Model file for the job. Use its own axes, mm. A direction names the side the tool comes from. Give positions to 0.01 mm unless a question says otherwise; leave off trailing zeros. Loops run counter-clockwise (first coordinate to the right, second up) from the corner with the lowest first, then second, coordinate; pieces in that order, holes last. Notation, with made-up numbers: (16, 1.25) - (39, 1.25) arc R20 ccw to (39, 31.25) - close; hole circle Ø7 at (0, 89). An arc over 180 degrees is marked (long way). Answer as CSV lines item,"result". Start each with the question number.
Item 1: Drill centre lines: L1, parallel to Y at x = 575, z = 109; L2, parallel to Z at x = 522.5, y = 36.5; L3, parallel to X at y = 82.5, z = 88. Where is each one in solid material? Low to high. Write a range as from..to.
Item 2: Pin check, flat tips, straight feed: pin 1 (5 mm diameter, centred on x = 640.5, z = 101.5, fed in from +Y); pin 2 (10 mm diameter, centred on y = 115.5, z = 57, fed in from -X); pin 3 (5 mm diameter, centred on y = 26.5, z = 36.5, fed in from +X). Stop position of each tip, or through.
Item 3: Saw through at D-D on y = 101.5. Give the cut face in (x, z), plus the area to 3 significant figures.
Item 4: Pull direction X, two halves, no side cores. Call faces 1 (the flat face through (609.33, 88.2, 59.16)), 2 (the flat face through (645, 94, 64)), 3 (the flat face through (591, 28, 130)): pulls with the +X half, pulls with the -X half, needs draft (parallel to the pull), parting line crosses it, or undercut.
Item 5: Saw through at B-B on z = 59. Give the cut face in (x, y), plus the area to 3 significant figures.
Item 6: Tool access for faces 4 (the flat face through (550, 50, 64)), 5 (the cylindrical face through (600.02, 0.88, 125.07)), 6 (the cylindrical face through (659.11, -8.4, 59.16)), 7 (the flat face through (588, 10, 120)): list every direction of +Z, -Z, +X, -X, +Y, -Y with a clear straight run to the whole face (end or side of a thin tool).
Item 7: Saw through at A-A on y = 0. Give the cut face in (x, z), plus the area to 3 significant figures.
Item 8: Saw through at C-C on x = 567. Give the cut face in (y, z), plus the area to 3 significant figures.
from build123d import *

# Parameters (mm, degrees)
EXTRUDE_1_DEPTH     = 130
SHELL_2_T           = -10
SKETCH_2_W          = 10
SKETCH_2_H          = 80.0247511
CUT_EXTRUDE_1_DEPTH = 120
SKETCH_3_R          = 20
CUT_EXTRUDE_2_DEPTH = 10


with BuildPart() as part:
    # 草图1 → 凸台-拉伸1 (new body)
    with BuildSketch(Plane.XY):
        with BuildLine():
            Line((574.017492235, -50), (620, -50))
            ThreePointArc((620, -50), (668.296291314, -12.940952255), (645, 43.301270189))
            Line((645, 43.301270189), (645, 145.857170879))
            ThreePointArc((645, 145.857170879), (632.507345261, 145.214355663), (620, 145))
            Line((620, 145), (584.288816548, 50))
            Line((584.288816548, 50), (514.017492235, 50))
            Line((514.017492235, 50), (514.017492235, 22.675903866))
            Line((514.017492235, 22.675903866), (514.017492235, -50.0247511))
            Line((514.017492235, -50.0247511), (573.94648172, -50.0247511))
            Line((573.94648172, -50.0247511), (574.017492235, -50))
        make_face()
    extrude(amount=EXTRUDE_1_DEPTH)

    # 抽壳2
    shell_2_openings = [part.faces().sort_by_distance(p)[0] for p in [
        (594.932550523, 20.025269894, 0),
    ]]
    offset(amount=SHELL_2_T, openings=shell_2_openings, kind=Kind.INTERSECTION)

    # 草图2 → 切除-拉伸1 (cut)
    with BuildSketch(Plane(origin=(0, 0, 0), x_dir=(-1, 0, 0), z_dir=(0, 0, -1))):
        with Locations((-519.017492235, -0.01237555)):
            Rectangle(SKETCH_2_W, SKETCH_2_H)
    extrude(amount=-CUT_EXTRUDE_1_DEPTH, mode=Mode.SUBTRACT)

    # 草图3 → 切除-拉伸2 (cut)
    with BuildSketch(Plane.XY.offset(130)):
        with Locations((620, 0)):
            Circle(SKETCH_3_R)
    extrude(amount=-CUT_EXTRUDE_2_DEPTH, mode=Mode.SUBTRACT)


solid = part.part
Responses:
1,L1,"-50..-40, 40..50"
1,L2,"120..130"
1,L3,"596.51..607.19, 635..645"
2,pin 1,"y = 145.73"
2,pin 2,"x = 607.03"
2,pin 3,"x = 663.86"
3,outline,"(603.65, 0) - (614.33, 0) - (614.33, 120) - (635, 120) - (635, 0) - (645, 0) - (645, 130) - (603.65, 130) - close"
3,area,"2,900 mm2"
4,face 1,"undercut"
4,face 2,"pulls with the +X half"
4,face 3,"needs draft"
5,outline,"(514.02, -50.02) - (573.95, -50.02) - (574.02, -50) - (620, -50) arc R50 ccw to (645, 43.3) - (645, 145.86) arc R365 cw to (620, 145) - (584.29, 50) - (514.02, 50) - (514.02, 40) - (591.21, 40) - (626.95, 135.06) arc R375 ccw to (635, 135.3) - (635, 37.08) arc R40 cw to (620, -40) - (572.32, -40) - (572.25, -40.02) - (514.02, -40.02) - close"
5,area,"5,190 mm2"
6,face 4,"+Z, -Z, -X, +Y"
6,face 5,"+Z, -Z"
6,face 6,"-Z, -X"
6,face 7,"-Z"
7,outline,"(514.02, 120) - (600, 120) - (600, 130) - (514.02, 130) - close; (640, 120) - (660, 120) - (660, 0) - (670, 0) - (670, 130) - (640, 130) - close"
7,area,"2,360 mm2"
8,outline,"(-50.02, 0) - (-40.02, 0) - (-40.02, 120) - (40, 120) - (40, 0) - (50, 0) - (50, 130) - (-50.02, 130) - close"
8,area,"3,400 mm2"
